Here's how the part is built. I have some questions about the finished solid (model axes, mm). Face numbers are marked on the shaded views. Round coordinates to 2 decimals unless told otherwise and drop trailing zeros. Write each loop counter-clockwise with the first axis right and the second up, starting at its lowest first coordinate (ties: lowest second). Pieces come first, ordered by that corner, then holes. Notation, with made-up numbers: (5, 5) -> (49, 5) arc R19 ccw to (49, 41) -> close; hole circle Ø7 at (-24.75, 88.25). An arc over 180 degrees is marked (long way). Answer as CSV lines item,"result".
from build123d import *

# Parameters (mm, degrees)
PAD_DEPTH    = 304.8
CHAMFER_SIZE = 254


with BuildPart() as part:
    # Sketch → Pad (new body)
    with BuildSketch(Plane.XY):
        Polygon((-806.45, -146.05), (-476.25, 365.125), (161.925, 266.7), (412.75, -15.875), align=None)
    extrude(amount=PAD_DEPTH)

    # Chamfer
    chamfer_edges = [part.edges().sort_by_distance(p)[0] for p in [
        (-196.85, -80.9625, 304.8),
    ]]
    chamfer(chamfer_edges, length=CHAMFER_SIZE)


solid = part.part
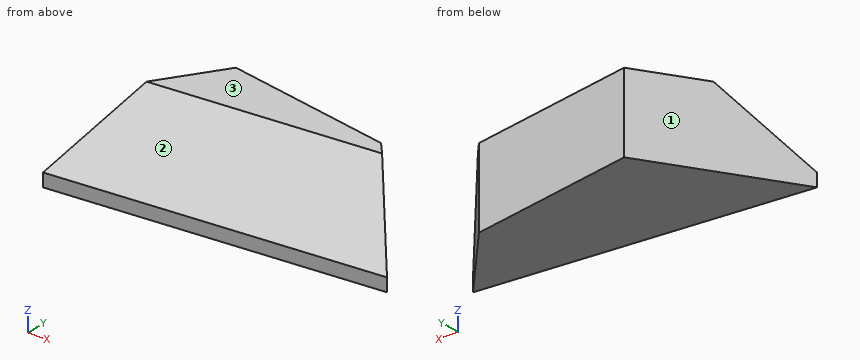
Item 1: If we mould it in two halves opening along X, with no side actions, what happens to the marked faces 1, 2 and 3? For each: pulls with the +X half, pulls with the -X half, needs draft (parallel to the pull), parting line crosses it, or undercut.
Results found:
face 1,"pulls with the -X half"
face 2,"pulls with the +X half"
face 3,"needs draft"
Item 2: Suppose I cut it at C-C, the plane z = 280. List the corners of the cut face in (x, y) for me (3 decimals).
Results found:
outline,"(-646.524, 101.528) -> (225.859, 194.673) -> (161.925, 266.7) -> (-476.25, 365.125) -> close"
Item 3: I need wall thicknesses on L1, parallel to X at y = 155, z = 186; L2, parallel to Y at x = -495, z = 145; L3, parallel to X at y = 141.5, z = 113. Which ranges of each line are inside material? Lowest first, please.
Results found:
L1,"x = -611.98 to 261.07"
L2,"y = -18.06 to 336.1"
L3,"x = -620.7 to 273.06"
Item 4: Suppose I cut it at A-A, the plane x = -365.5. List the corners of the cut face in (y, z) for me.
Results found:
outline,"(-98.97, 0) -> (348.04, 0) -> (348.04, 304.8) -> (156.47, 304.8) -> (-98.97, 50.8) -> close"
Item 5: Will these pins go through, and if not, where does the flat tip stop? pin 1 (1 mm diameter, centred on x = 47, y = 133.5, fed in from +Z); pin 2 (12 mm diameter, centred on x = 65.5, y = 49.5, fed in from -Z); pin 3 (4 mm diameter, centred on y = 107.5, z = 142, fed in from +X); pin 4 (1 mm diameter, centred on x = -174, z = 236, fed in from +Y).
Results found:
pin 1,"stops at z = 238.66"
pin 2,"stops at z = 0"
pin 3,"stops at x = 305.01"
pin 4,"stops at y = 318.59"
Item 6: Suppose I cut it at B-B, the plane y = -99.5. List the corners of the cut face in (x, z) for me.
Results found:
outline,"(-776.38, 0) -> (-370.47, 0) -> (-370.47, 50.8) -> (-776.38, 93.89) -> close"
Item 7: Suppose I cut it at D-D, the plane x = -224.5. List the corners of the cut face in (y, z) for me, then the cut area to 3 significant figures.
Results found:
outline,"(-83.91, 0) -> (326.3, 0) -> (326.3, 304.8) -> (171.53, 304.8) -> (-83.91, 50.8) -> close"
area,"92,600 mm²"
